The listing builds one solid part. Answer for the finished solid, in the listing's coordinates (mm). A direction names the side the tool comes from. Give positions to 0.01 mm unless a question says otherwise; leave off trailing zeros. Write each loop counter-clockwise with the first axis right and the second up, starting at its lowest first coordinate (ties: lowest second). Pieces come first, ordered by that corner, then holes. Notation, with made-up numbers: M 5.5,7 L 63.5,7 A15 cw 63.5,25 Z; hole C 76.5,72.5 d11. An arc over 180 degrees is marked long. Return JSON: item names as keys, results as strings.
from build123d import *

# Parameters (mm, degrees)
SKETCH1_R           = 25
BOSS_EXTRUDE1_DEPTH = 4.5
SKETCH2_R           = 12
BOSS_EXTRUDE2_DEPTH = 13
SKETCH3_R           = 7
CUT_EXTRUDE1_DEPTH  = 17.5
SKETCH4_R           = 2.5
CUT_EXTRUDE2_DEPTH  = 4.5
SKETCH5_R           = 2.5
CUT_EXTRUDE3_DEPTH  = 25


with BuildPart() as part:
    # Sketch1 → Boss-Extrude1 (new body)
    with BuildSketch(Plane(origin=(0, 0, 0), x_dir=(1, 0, 0), z_dir=(0, 1, 0))):
        Circle(SKETCH1_R)
    extrude(amount=BOSS_EXTRUDE1_DEPTH)

    # Sketch2 → Boss-Extrude2 (add)
    with BuildSketch(Plane(origin=(0, 4.5, 0), x_dir=(1, 0, 0), z_dir=(0, 1, 0))):
        Circle(SKETCH2_R)
    extrude(amount=BOSS_EXTRUDE2_DEPTH)

    # Sketch3 → Cut-Extrude1 (cut)
    with BuildSketch(Plane(origin=(0, 17.5, 0), x_dir=(1, 0, 0), z_dir=(0, 1, 0))):
        Circle(SKETCH3_R)
    extrude(amount=-CUT_EXTRUDE1_DEPTH, mode=Mode.SUBTRACT)

    # Sketch4 → Cut-Extrude2 (cut)
    with BuildSketch(Plane(origin=(0, 4.5, 0), x_dir=(1, 0, 0), z_dir=(0, 1, 0))):
        with Locations((-18.5, 0)):
            Circle(SKETCH4_R)
        with Locations((0, 18.5)):
            Circle(SKETCH4_R)
        with Locations((18.5, 0)):
            Circle(SKETCH4_R)
        with Locations((0, -18.5)):
            Circle(SKETCH4_R)
    extrude(amount=-CUT_EXTRUDE2_DEPTH, mode=Mode.SUBTRACT)

    # Sketch5 → Cut-Extrude3 (cut)
    with BuildSketch(Plane(origin=(0, 0, 0), x_dir=(0, 0, -1), z_dir=(1, 0, 0))):
        with Locations((0, 11)):
            Circle(SKETCH5_R)
    extrude(amount=-CUT_EXTRUDE3_DEPTH, mode=Mode.SUBTRACT)


solid = part.part
Item 1: Find the intervals of material crossed by line 1 (Z direction, x = 0, y = 2.2); line 2 (Y direction, x = -9.6, z = 0), in increasing order.
Geometry results:
{"line 1": "z = -25 to -21, -16 to -7, 7 to 16, 21 to 25", "line 2": "y = 0 to 8.5, 13.5 to 17.5"}
Item 2: Determine the mould class of faces 1 (the cylindrical face through (11.446, 10.909, -3.604)), 2 (the flat face through (5.2, 17.5, 5.2)), 3 (the cylindrical face through (6.677, 8.872, -2.103)) for opening direction X: +X half, -X half, draft (parallel to the pull), parting line (faces both ways), or undercut.
Geometry results:
{"face 1": "parting line", "face 2": "draft", "face 3": "undercut"}
Item 3: Which of the six approach directions +Z, -Z, +X, -X, +Y, -Y give full straight-line access (tool end or side, diameter ignored) to faces 4 (the cylindrical face through (-9.2, 11.1, 2.5)), 5 (the flat face through (5.2, 0, 5.2)), 6 (the flat face through (-6, 4.5, 11))?
Geometry results:
{"face 4": "-X", "face 5": "+Z, -Z, +X, -X, -Y", "face 6": "+Y"}
Item 4: A cutting plane is placed at C-C, the plane y = 2. Write down the section's boundary in (x, z), plus the area to 3 significant figures.
Geometry results:
{"outline": "C 0,0 d50; hole C -18.5,0 d5; hole C 0,0 d14; hole C 0,-18.5 d5; hole C 0,18.5 d5; hole C 18.5,0 d5", "area": "1,730 mm2"}
Item 5: A cutting plane is placed at A-A, the plane z = 20. Write down the section's boundary in (x, y), plus the area to 3 significant figures.
Geometry results:
{"outline": "M -15,0 L -2,0 L -2,4.5 L -15,4.5 Z; M 2,0 L 15,0 L 15,4.5 L 2,4.5 Z", "area": "117 mm2"}
Item 6: Given pin 1 Ø4 at (x, y) = (-2, 11) entering from +Z; pin 2 Ø12 at (x, z) = (-16.5, -13.5) entering from +Y; pin 3 Ø6 at (x, y) = (5.5, 10) entering from +Z; pin 4 Ø11 at (x, z) = (0, 0) entering from -Y, each flat-ended and moving along its own axis, determine where each tip first touches the part or whether it passes through.
Geometry results:
{"pin 1": "stops at z = 12", "pin 2": "stops at y = 4.5", "pin 3": "stops at z = 11.74", "pin 4": "passes through"}
Item 7: A cutting plane is placed at D-D, the plane x = 5. Write down the section's boundary in (y, z), plus the area to 3 significant figures.
Geometry results:
{"outline": "M 0,-24.49 L 4.5,-24.49 L 4.5,-10.91 L 17.5,-10.91 L 17.5,-4.9 L 0,-4.9 Z; M 0,4.9 L 17.5,4.9 L 17.5,10.91 L 4.5,10.91 L 4.5,24.49 L 0,24.49 Z", "area": "333 mm2"}
Item 8: A cutting plane is placed at B-B, the plane x = 0. Write down the section's boundary in (y, z), plus the area to 3 significant figures.
Geometry results:
{"outline": "M 0,-25 L 4.5,-25 L 4.5,-21 L 0,-21 Z; M 0,-16 L 4.5,-16 L 4.5,-12 L 17.5,-12 L 17.5,-7 L 0,-7 Z; M 0,7 L 17.5,7 L 17.5,12 L 4.5,12 L 4.5,16 L 0,16 Z; M 0,21 L 4.5,21 L 4.5,25 L 0,25 Z", "area": "247 mm2"}
